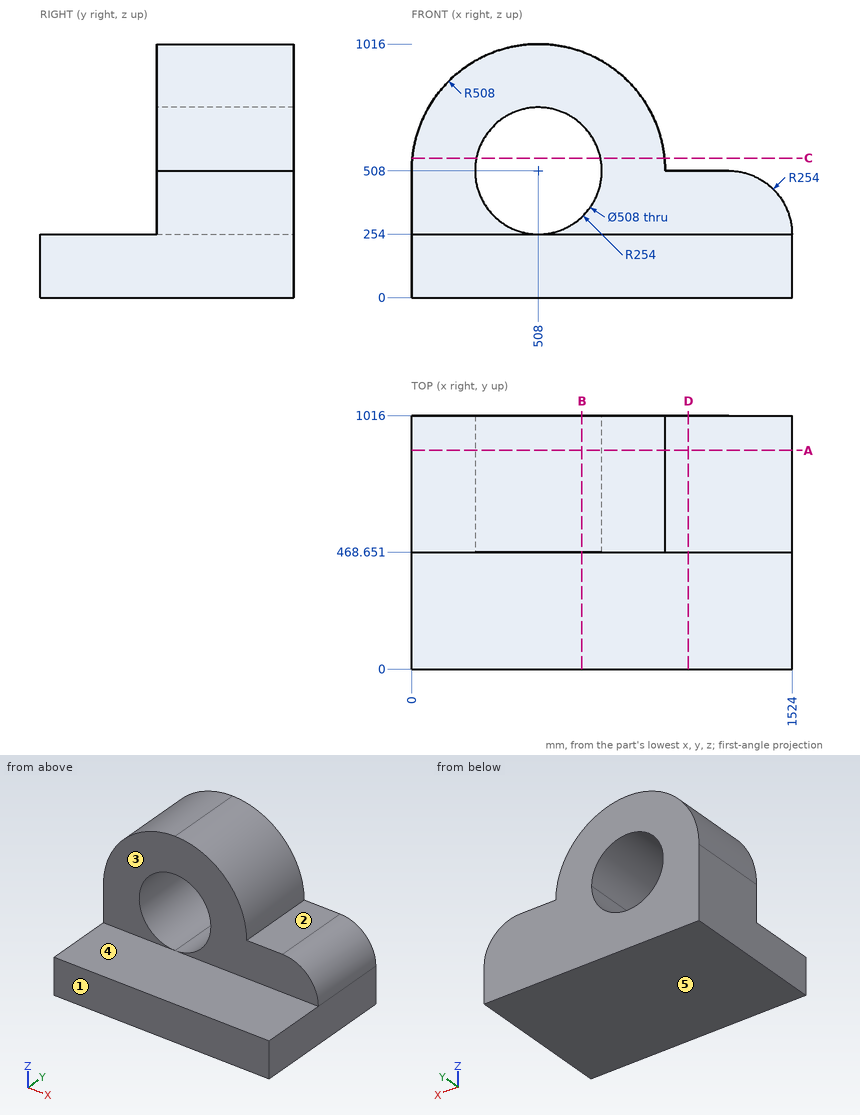
Check sheet for the drawn part. Datum: minimum x, y, z corner. Units: mm. A direction names the side the tool comes from. Coordinates: 2 decimals unless noted, no trailing zeros. Loops run counter-clockwise (first coordinate to the right, second up) from the corner with the lowest first, then second, coordinate; pieces in that order, holes last. Notation, with made-up numbers: (15.25, -33.5) -> (46.25, -33.5) arc R9 cw to (46.25, -29.5) -> close; hole circle Ø8 at (8, 5). An arc over 180 degrees is marked (long way). Answer as CSV lines item,"result".
1) Cross-section at A-A, the plane y = 877. Record the cut outline in (x, z).
Found:
outline,"(0, 0) -> (1524, 0) -> (1524, 254) arc R254 ccw to (1270, 508) -> (1016, 508) arc R508 ccw to (508, 1016) arc R508 ccw to (0, 508) -> close; hole (508, 254) arc R254 ccw to (762, 508) arc R254 ccw (long way) to start"
2) Cross-section at D-D, the plane x = 1109. Record the cut outline in (y, z).
Found:
outline,"(0, 0) -> (1016, 0) -> (1016, 508) -> (468.65, 508) -> (468.65, 254) -> (0, 254) -> close"
3) Thickness scan on L1, parallel to Z at x = 508, y = 834.5; L2, parallel to Y at x = 871.5, z = 327; L3, parallel to Z at x = 1280, y = 473.5. Record the ranges inside material, lowest first. Write a range as from..to.
Found:
L1,"z = 0..254, 762..1016"
L2,"y = 468.65..1016"
L3,"z = 0..507.8"
4) Depth check by flat-ended pin: pin 1 (3 mm diameter, centred on x = 188.5, z = 719, fed in from -Y); pin 2 (8 mm diameter, centred on y = 742.5, z = 554, fed in from +X); pin 3 (4 mm diameter, centred on x = 299.5, y = 236, fed in from +Z). Enter the tip coordinate at first touch or a pass-through.
Found:
pin 1,"stops at y = 468.65"
pin 2,"stops at x = 1014.26"
pin 3,"stops at z = 254"
5) Release check for a two-part mould opening along Z. For the marked faces 3, 4 and 5 record: +Z half, -Z half, draft (parallel to the pull), parting line (faces both ways), or undercut.
Found:
face 3,"draft"
face 4,"+Z half"
face 5,"-Z half"
6) Tool access check on the marked faces 1 and 2. Record the directions out of +Z, -Z, +X, -X, +Y, -Y that give a thin tool (end or side, any length) a straight path to the whole face; none if there is none.
Found:
face 1,"+Z, -Z, +X, -X, -Y"
face 2,"+Z, +X, +Y, -Y"
7) Cross-section at B-B, the plane x = 682. Record the cut outline in (y, z).
Found:
outline,"(0, 0) -> (1016, 0) -> (1016, 322.96) -> (468.65, 322.96) -> (468.65, 254) -> (0, 254) -> close; (468.65, 693.04) -> (1016, 693.04) -> (1016, 985.27) -> (468.65, 985.27) -> close"
8) Cross-section at C-C, the plane z = 558.5. Record the cut outline in (x, y).
Found:
outline,"(2.52, 468.65) -> (259.07, 468.65) -> (259.07, 1016) -> (2.52, 1016) -> close; (756.93, 468.65) -> (1013.48, 468.65) -> (1013.48, 1016) -> (756.93, 1016) -> close"
